Autodesk Inventor part; units mm, degrees
ref_plane "YZ Plane" through (0, 0, 0) normal (1, 0, 0) x (0, 1, 0)
ref_plane "XZ Plane" through (0, 0, 0) normal (0, 1, 0) x (-1, 0, 0)
ref_plane "XY Plane" through (0, 0, 0) normal (0, 0, 1) x (1, 0, 0)
sketch "Sketch55" plane through (0, 0, 0) normal (0, 0, 1) x (1, 0, 0)
  line L0 (0, 0) -> (0, -53.4597) construction
  line L1 (0, 0) -> (31.8198, 31.8198)
  line L2 (0, 0) -> (89.157, 0) construction
  line L3 (0, 0) -> (-31.8198, -31.8198)
  line L4 (31.8198, 31.8198) -> (-31.8198, 31.8198)
  line L5 (-31.8198, 31.8198) -> (-31.8198, -31.8198)
  dimension "d252" = 45
extrude "Extrusion25" add sketch "Sketch55" along normal mid plane 150
sketch "Sketch56" plane through (-31.8198, 31.8198, 75) normal (0, 1, 0) x (1, 0, 0)
  line L0 (0, 150) -> (63.6396, 150)
  line L1 (63.6396, 0) -> (63.6396, 150)
  line L2 (0, 150) -> (0, 0)
  line L3 (63.6396, 0) -> (0, 0)
  line L4 (0, 150) -> (63.6396, 150)
  line L5 (63.6396, 150) -> (63.6396, 0)
  line L6 (63.6396, 0) -> (0, 0)
  line L7 (0, 0) -> (0, 150)
  point P0 (31.8198, 75)
extrude "Extrusion26" add sketch "Sketch56" along normal blind 50
sketch "Sketch57" plane through (-31.8198, 81.8198, 75) normal (0, 1, 0) x (1, 0, 0)
  line L0 (63.6396, 150) -> (0, 150)
  line L1 (63.6396, 0) -> (63.6396, 150)
  line L2 (0, 0) -> (63.6396, 0)
  line L3 (0, 150) -> (0, 0)
  line L4 (0, 54.68) -> (63.6396, 54.68)
  line L5 (63.6396, 54.68) -> (63.6396, 95.32)
  line L6 (63.6396, 95.32) -> (0, 95.32)
  line L7 (0, 95.32) -> (0, 54.68)
  line L8 (0, 54.68) -> (63.6396, 95.32) construction
  line L9 (63.6396, 54.68) -> (0, 95.32) construction
  line L10 (0, 95.32) -> (63.6396, 95.32)
  line L11 (63.6396, 95.32) -> (63.6396, 103.42)
  line L12 (63.6396, 103.42) -> (0, 103.42)
  line L13 (0, 103.42) -> (0, 95.32)
  line L14 (0, 54.68) -> (63.6396, 54.68)
  line L15 (63.6396, 54.68) -> (63.6396, 46.58)
  line L16 (63.6396, 46.58) -> (0, 46.58)
  line L17 (0, 46.58) -> (0, 54.68)
  point P0 (31.8198, 75)
  point P1 (0, 46.58)
  point P2 (0, 103.42)
  point P3 (0, 95.32)
  dimension "d259" = 8.1
  dimension "d260" = 8.1
  dimension "d261" = 40.64
extrude "Extrusion27" add sketch "Sketch57" along normal blind 101.6 contours L1 L6 L3 L12 | L1 L16 L3 L4
equation "\"d261\" = twoByFourWidth"
equation "\"wallThickness\" = 8"
equation "\"twoByFourWidth\" = 40.64"
equation "\"twoByFourDepth\" = 84.1375"
equation "\"azimuth\" = -15deg"
equation "\"elevation\" = 20deg"
equation "\"depthOfExtrusionForMatingToLowerHalf\" = 12.5"
equation "\"depthForWasherForMatingToCase\" = 14"
equation "\"topWallThickness\" = 8"
equation "\"widthOfCase\" = 149"
equation "\"sideWallThickness\" = 8"
equation "\"caseHeight\" = 125"
equation "\"bottomWallThickness\" = 8"
properties part number "upperBracketForSquareBracket" material "PC/ABS Plastic"
Here's how the part is built. I have some questions about the finished solid (model axes, mm). A direction names the side the tool comes from. Coordinates: 2 decimals unless noted, no trailing zeros. Write each loop counter-clockwise with the first axis right and the second up, starting at its lowest first coordinate (ties: lowest second). Pieces come first, ordered by that corner, then holes. Notation, with made-up numbers: (-35.5, 36) -> (-17.5, 36) arc R28 ccw to (-17.5, 55) -> close; hole circle Ø10 at (65, 84). An arc over 180 degrees is marked (long way). Use a Markdown table: item, result. Add a question column.
(1) We'd pull the mould along Z, two halves only. Please class faces 4 (the flat face through (0, 81.82, 0)), 5 (the flat face through (0, 132, -28.42)), 6 (the flat face through (0, 183.42, 24)), 7 (the flat face through (0, 132, 28.42)): +Z half, -Z half, draft (parallel to the pull), parting line (faces both ways), or undercut.
(2) If we section it at A-A, the plane y = 106.5: Write out the boundary of the cut face in (x, z), and give its area (3 significant figures).
(3) If we section it at B-B, the plane x = -14: Write out the boundary of the cut face in (y, z).
(4) If we section it at C-C, the plane z = 3: Write out the boundary of the cut face in (x, y).
(5) I'm going to push flat-ended pins straight in: P1, Ø4, axis at x = 11, z = 53.5, coming from the -Y side; P2, Ø14, axis at x = -13.5, z = 56, coming from the +Y side; P3, Ø8, axis at x = 17.5, y = 153.5, coming from the -Z side; P4, Ø12, axis at x = 21, y = 8, coming from the +Z side. Where does each tip first touch, or does it pass through?
(6) For faces 1 (the flat face through (0, 81.82, 51)), 2 (the flat face through (0, 132, 20.32)), 3 (the flat face through (0, 81.82, -52)), which set-ups out of +Z, -Z, +X, -X, +Y, -Y let a thin tool reach every point of the face, with its end or its side?
(7) If we section it at D-D, the plane y = 1: Write out the boundary of the cut face in (x, z), and give its area (3 significant figures).
(8) Please list where these lines run through material, in increasing order: line 1 (Z direction, x = 16, y = 94); line 2 (Y direction, x = 4.5, z = -11.5); line 3 (Y direction, x = -4, z = 41).
Outcome:
| question | item | result |
|---|---|---|
| 1 | face 4 | undercut |
| 1 | face 5 | -Z half |
| 1 | face 6 | draft |
| 1 | face 7 | +Z half |
| 2 | outline | (-31.82, -28.42) -> (31.82, -28.42) -> (31.82, -20.32) -> (-31.82, -20.32) -> close; (-31.82, 20.32) -> (31.82, 20.32) -> (31.82, 28.42) -> (-31.82, 28.42) -> close |
| 2 | area | 1,030 mm^2 |
| 3 | outline | (-14, -75) -> (81.82, -75) -> (81.82, -28.42) -> (183.42, -28.42) -> (183.42, -20.32) -> (81.82, -20.32) -> (81.82, 20.32) -> (183.42, 20.32) -> (183.42, 28.42) -> (81.82, 28.42) -> (81.82, 75) -> (-14, 75) -> close |
| 4 | outline | (-31.82, -31.82) -> (31.82, 31.82) -> (31.82, 81.82) -> (-31.82, 81.82) -> close |
| 5 | P1 | stops at y = 9 |
| 5 | P2 | stops at y = 81.82 |
| 5 | P3 | stops at z = -28.42 |
| 5 | P4 | passes through |
| 6 | face 1 | +Z, +X, -X, +Y |
| 6 | face 2 | +X, -X, +Y |
| 6 | face 3 | -Z, +X, -X, +Y |
| 7 | outline | (-31.82, -75) -> (1, -75) -> (1, 75) -> (-31.82, 75) -> close |
| 7 | area | 4,920 mm^2 |
| 8 | line 1 | z = -28.42 to -20.32, 20.32 to 28.42 |
| 8 | line 2 | y = 4.5 to 81.82 |
| 8 | line 3 | y = -4 to 81.82 |
